```python
from build123d import *

# Parameters (mm, degrees)
EXTRUDE_1_DEPTH     = 1
SKETCH_2_R          = 1.5
CUT_EXTRUDE_1_DEPTH = 10


with BuildPart() as part:
    # 草图1 → 凸台-拉伸1 (new, symmetric)
    with BuildSketch(Plane.XY):
        with BuildLine():
            ThreePointArc((109, 0), (0, 109), (-109, 0))
            Line((-109, 0), (-65, 0))
            Line((-65, 0), (-65, 65))
            Line((-65, 65), (65, 65))
            Line((65, 65), (65, 0))
            Line((65, 0), (109, 0))
        make_face()
    extrude(amount=EXTRUDE_1_DEPTH, both=True)

    # 草图2 → 切除-拉伸1 (cut)
    with BuildSketch(Plane.XY.offset(1)):
        with Locations((44, 68)):
            Circle(SKETCH_2_R)
        with Locations((24, 68)):
            Circle(SKETCH_2_R)
        with Locations((-30, 68)):
            Circle(SKETCH_2_R)
        with Locations((-50, 68)):
            Circle(SKETCH_2_R)
    extrude(amount=-CUT_EXTRUDE_1_DEPTH, mode=Mode.SUBTRACT)


solid = part.part
```
Check sheet for the modelled part. Datum: model origin and axes. Units: mm. Coordinates: 2 decimals unless noted, no trailing zeros. Order: outer loops, then holes, each group sorted by start corner. A loop starts at its lowest first (then second) coordinate and runs counter-clockwise, first axis right, second up. Notation, with made-up numbers: M 67.25,-18 L 75.25,-18 A16 ccw 75.25,9 Z; hole C 10,23 d10. An arc over 180 degrees is marked long. One line per question, with ' | ' between items. Start each with the question number.
Item 1: Material ranges on line 1 (X direction, y = 68, z = -0.5); line 2 (X direction, y = 51, z = 0.1); line 3 (X direction, y = 64.5, z = -0.55), recorded low to high.
Item 2: Gauge pin test, flat ends, axial feed: P1, Ø0.6, axis at y = 16.5, z = 0, coming from the +X side; P2, Ø3.5, axis at x = 44, y = 68, coming from the +Z side; P3, Ø1.8, axis at x = -50, y = 68, coming from the +Z side. Record the tip position at first contact, or that the pin passes through.
Item 3: Sectioned sample at B-B on x = 0. Record the cut outline in (y, z).
Item 4: Sectioned sample at A-A on z = 0.7. Record the cut outline in (x, y), and give its area (3 significant figures).
Item 5: Sectioned sample at C-C on y = 76. Record the cut outline in (x, z).
Answer below:
1) line 1: x = -85.19 to -51.5, -48.5 to -31.5, -28.5 to 22.5, 25.5 to 42.5, 45.5 to 85.19 | line 2: x = -96.33 to -65, 65 to 96.33 | line 3: x = -87.87 to -65, 65 to 87.87
2) P1: stops at x = 107.79 | P2: stops at z = 1 | P3: passes through
3) outline: M 65,-1 L 109,-1 L 109,1 L 65,1 Z
4) outline: M -109,0 L -65,0 L -65,65 L 65,65 L 65,0 L 109,0 A109 ccw Z; hole C -50,68 d3; hole C -30,68 d3; hole C 24,68 d3; hole C 44,68 d3 | area: 10,200 mm^2
5) outline: M -78.13,-1 L 78.13,-1 L 78.13,1 L -78.13,1 Z
